Source: CAD feature listing. Evaluate the final solid. Frame: model axes, mm. Face numbers are marked on the shaded views. A direction names the side the tool comes from. Give positions to 0.01 mm unless a question says otherwise; leave off trailing zeros. Order: outer loops, then holes, each group sorted by start corner. A loop starts at its lowest first (then second) coordinate and runs counter-clockwise, first axis right, second up. Notation, with made-up numbers: (-6.5, 71.25) - (20.5, 71.25) arc R29 ccw to (20.5, 107.25) - close; hole circle Ø7 at (-10, -23.75). An arc over 180 degrees is marked (long way). Write each question's results on one line, items separated by ' | '. Start each with the question number.
Item 1: Section C-C on y = -3.5. Output: boundary loops of the cut face in (x, z), and give its area (3 significant figures).
Item 2: Section B-B on x = -9. Output: boundary loops of the cut face in (y, z).
Item 3: Line query: line 1 along Y through (x, z) = (-73.4, -0.1); line 2 along Z through (x, y) = (-23.5, 0.25); line 3 along Z through (x, y) = (-45, 1.75). Output: solid intervals per line, ascending.
Item 4: Section A-A on x = -62.5. Output: boundary loops of the cut face in (y, z).
Item 5: Set-up query: the marked faces 1 and 2. Return all of +Z, -Z, +X, -X, +Y, -Y with unobstructed straight access to the full face (end or side cutting, diameter ignored); none if empty.
Item 6: Contact query for flat-ended pins moving along their axis: pin 1 Ø1.6 at (x, y) = (-73.4, -10) entering from +Z; pin 2 Ø0.6 at (x, y) = (-31.5, 1.5) entering from +Z; pin 3 Ø1 at (y, z) = (-4.5, 0.5) entering from +X. Output: stop coordinate, or through.
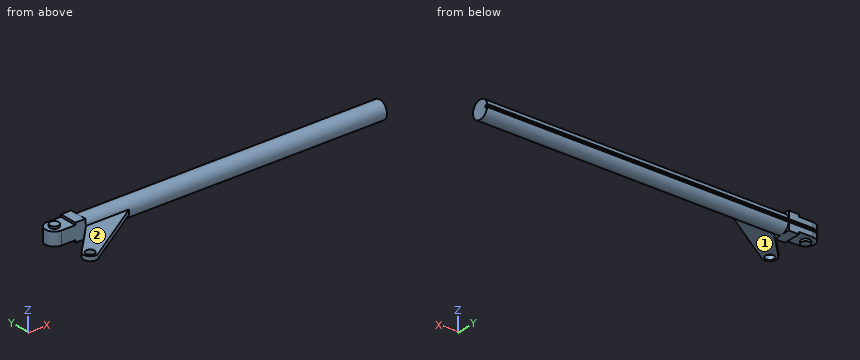
```python
from build123d import *

# Parameters (mm, degrees)
SKETCH_1_R               = 2
EXTRUDE_1_DEPTH          = 68
EXTRUDE_2_DEPTH          = 2
SKETCH_3_W               = 5.1
SKETCH_3_H               = 0.5
CUT_EXTRUDE_1_DEPTH      = 3
CUT_EXTRUDE_1_DEPTH_BACK = 3
SKETCH_4_R               = 1
EXTRUDE_3_DEPTH          = 2
SKETCH_5_W               = 75.4
SKETCH_5_H               = 0.6
CUT_EXTRUDE_2_DEPTH      = 0.5
SKETCH_6_R               = 1
EXTRUDE_4_DEPTH          = 0.5


with BuildPart() as part:
    # 草图1 → 凸台-拉伸1 (new body)
    with BuildSketch(Plane(origin=(0, 0, 0), x_dir=(0, 0, -1), z_dir=(1, 0, 0))):
        Circle(SKETCH_1_R)
    extrude(amount=-EXTRUDE_1_DEPTH)

    # 草图2 → 凸台-拉伸2 (add, symmetric)
    with BuildSketch(Plane.XY):
        with BuildLine():
            Line((-68, 2), (-73.4, 2))
            ThreePointArc((-73.4, 2), (-75.4, 0), (-73.4, -2))
            Line((-73.4, -2), (-68, -2))
            Line((-68, -2), (-68, 2))
        make_face()
    extrude(amount=EXTRUDE_2_DEPTH, both=True)

    # 草图3 → 切除-拉伸1 (cut, two sides)
    with BuildSketch(Plane(origin=(0, 0, 0), x_dir=(1, 0, 0), z_dir=(0, 1, 0))) as cut_extrude_1_sk:
        with Locations((-72.85, 1.75)):
            Rectangle(SKETCH_3_W, SKETCH_3_H)
        with Locations((-72.85, -1.75)):
            Rectangle(SKETCH_3_W, SKETCH_3_H)
    extrude(amount=CUT_EXTRUDE_1_DEPTH, mode=Mode.SUBTRACT)
    extrude(cut_extrude_1_sk.sketch, amount=-CUT_EXTRUDE_1_DEPTH_BACK, mode=Mode.SUBTRACT)

    # 草图4 → 凸台-拉伸3 (add, symmetric)
    with BuildSketch(Plane.XY):
        with Locations((-73.4, 0)):
            Circle(SKETCH_4_R)
    extrude(amount=EXTRUDE_3_DEPTH, both=True)

    # 草图5 → 切除-拉伸2 (cut)
    with BuildSketch(Plane(origin=(0, 2, 0), x_dir=(1, 0, 0), z_dir=(0, 1, 0))):
        with Locations((-37.7, 0)):
            Rectangle(SKETCH_5_W, SKETCH_5_H)
    extrude(amount=-CUT_EXTRUDE_2_DEPTH, mode=Mode.SUBTRACT)

    # 草图6 → 凸台-拉伸4 (add, symmetric)
    with BuildSketch(Plane.XY):
        with BuildLine():
            Line((-67.4, -1.5), (-57.4, -1.5))
            Line((-57.4, -1.5), (-72.589010682, -11.261862245))
            ThreePointArc((-72.589010682, -11.261862245), (-74.555588863, -10.956354736), (-74.487937961, -8.96733791))
            Line((-74.487937961, -8.96733791), (-67.4, -1.5))
        make_face()
        with Locations((-73.4, -10)):
            Circle(SKETCH_6_R, mode=Mode.SUBTRACT)
    extrude(amount=EXTRUDE_4_DEPTH, both=True)


solid = part.part
```
Evaluation:
1) outline: (-69.3, -0.5) - (-60.51, -0.5) - (-60.51, 0.5) - (-69.3, 0.5) - close | area: 8.79 mm^2
2) outline: (1.5, -0.3) - (1.5, 0.3) - (1.98, 0.3) arc R2 ccw (long way) to (1.98, -0.3) - close
3) line 1: y = -11.5 to -11, -9 to -7.82, -2 to 1.5 | line 2: z = -1.98 to 1.98 | line 3: z = -0.97 to -0.3, 0.3 to 0.97
4) outline: (-4.78, -0.5) - (-1.94, -0.5) arc R2 ccw to (1.98, -0.3) - (1.5, -0.3) - (1.5, 0.3) - (1.98, 0.3) arc R2 ccw to (-1.94, 0.5) - (-4.78, 0.5) - close
5) face 1: -Z, +X, -X, -Y | face 2: +Z, +X, -X, -Y
6) pin 1: passes through | pin 2: stops at z = 1.6 | pin 3: stops at x = -61.29
